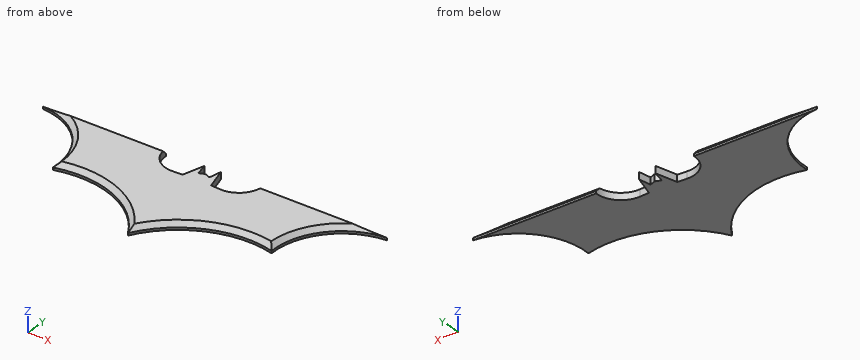
```python
from build123d import *

# Parameters (mm, degrees)
PAD_DEPTH    = 3
CHAMFER_SIZE = 2


with BuildPart() as body:
    # Sketch → Pad (new body)
    with BuildSketch(Plane.XY):
        with BuildLine():
            Line((0, 0), (0, 14.502488))
            Line((0, 14.502488), (2.444644, 13.541802))
            Line((2.444644, 13.541802), (3.525413, 18.825575))
            Line((3.525413, 18.825575), (6.167308, 9.459041))
            Line((6.167308, 9.459041), (10.250262, 9.218303))
            ThreePointArc((10.250262, 9.218303), (18.202038, 12.211905), (21.296978, 20.124789))
            Line((21.296978, 20.124789), (75, 20.124789))
            ThreePointArc((75, 20.124789), (54.90279, 10.195186), (47.700768, -11.032761))
            ThreePointArc((47.700768, -11.032761), (20.35465, -12.880568), (0, -31.235753))
            Line((0, -31.235753), (0, 0))
        make_face()
    extrude(amount=PAD_DEPTH)

    # Chamfer
    chamfer_edges = [body.edges().sort_by_distance(p)[0] for p in [
        (20.35465, -12.880568, 3),
        (54.90279, 10.195186, 3),
        (48.148489, 20.124789, 3),
    ]]
    chamfer(chamfer_edges, length=CHAMFER_SIZE)


with BuildPart() as part_mirroring:
    # Part__Mirroring: instance of Body
    add(body.part.mirror(Plane(origin=(0, 0, 0), x_dir=(0, -1, 0), z_dir=(1, 0, 0))))


with BuildPart() as fusion:
    # Fusion base: copy of Body
    add(body.part)

    # Fusion: union Part__Mirroring
    add(part_mirroring.part)


solid = fusion.part
```
Geometry: final body of the model. Coordinates: model frame, mm. Coordinates: 2 decimals unless noted, no trailing zeros. Write each loop counter-clockwise with the first axis right and the second up, starting at its lowest first coordinate (ties: lowest second). Pieces come first, ordered by that corner, then holes. Notation, with made-up numbers: M -10.75,78.25 L 5.25,78.25 A16 ccw 5.25,87.25 Z; hole C 65,-10 d1. An arc over 180 degrees is marked long. Use CSV: the item, a comma, the result in double quotes. Start each with the question number.
1. First-contact query: P1, Ø1, axis at y = 3, z = 2.5, coming from the +X side. Flat tip, straight axial feed; report the tip coordinate or a pass-through.
2. Cut plane A-A on y = 11. Count the separate pieces of the cut face and the enclosed holes in it, plus the area to 3 significant figures.
3. Ray query, probe 1 along Z at (x, y) = (-47, 0); probe 2 along Y at (x, z) = (-36, 0.75); probe 3 along X at (y, z) = (-4, 2). Return the intervals inside material, ascending.
4. Cut plane B-B on z = 1.5. Return the cut outline in (x, y), plus the area to 3 significant figures.
Entries:
1,P1,"x = 49.21"
2,separate pieces,"3"
2,enclosed holes,"0"
2,area,"262 mm²"
3,probe 1,"0 to 3"
3,probe 2,"-9.57 to 20.12"
3,probe 3,"-47.07 to 47.07"
4,outline,"M -69.05,19.62 A29.81 cw -47.16,-10.37 A42.4 cw 0,-30.22 A42.4 cw 47.16,-10.37 A29.81 cw 69.05,19.62 L 21.31,19.62 A10.44 cw 10.25,9.22 L 6.17,9.46 L 3.53,18.83 L 2.44,13.54 L 0,14.5 L -2.44,13.54 L -3.53,18.83 L -6.17,9.46 L -10.25,9.22 A10.44 cw -21.31,19.62 Z"
4,area,"3,160 mm²"
